Could you check a few things on this model? Use its own coordinates, in mm. Face numbers are marked on the shaded views. A direction names the side the tool comes from. Give positions to 0.01 mm unless a question says otherwise; leave off trailing zeros. Loops run counter-clockwise (first coordinate to the right, second up) from the corner with the lowest first, then second, coordinate; pieces in that order, holes last. Notation, with made-up numbers: (-14.75, -20) - (30.25, -20) arc R24 cw to (30.25, -3) - close; hole circle Ø11 at (-29, 60). An arc over 180 degrees is marked (long way). Use CSV: the item, a comma, the result in double quotes.
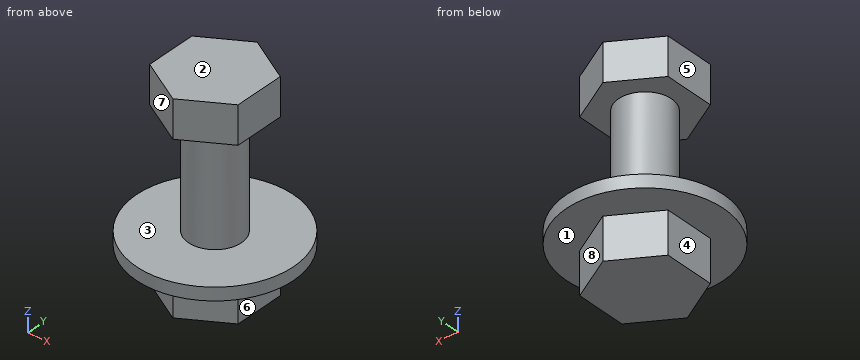
from build123d import *

# Parameters (mm, degrees)
F0_R     = 3
F1_DEPTH = 20
F3_DEPTH = 4.24
F5_DEPTH = 6
F6_R     = 8.89
F7_DEPTH = 1.4478
F9_DEPTH = 1.27


with BuildPart() as f1:
    # F0 (on Top) → F1 (new body)
    with BuildSketch(Plane.XY):
        Circle(F0_R)
    extrude(amount=-F1_DEPTH)

    # F2 (on face) → F3 (join)
    with BuildSketch(Plane.XY):
        Polygon((5, 2.8867513459), (0, 5.7735026919), (-5, 2.8867513459), (-5, -2.8867513459), (0, -5.7735026919), (5, -2.8867513459), align=None)
    extrude(amount=F3_DEPTH)

    # F4 (on face) → F5 (join)
    with BuildSketch(Plane(origin=(0, 0, -20), x_dir=(1, 0, 0), z_dir=(0, 0, -1))):
        Polygon((5, 2.8867513459), (0, 5.7735026919), (-5, 2.8867513459), (-5, -2.8867513459), (0, -5.7735026919), (5, -2.8867513459), align=None)
    extrude(amount=-F5_DEPTH)

    # F6 (on face) → F7 (join)
    with BuildSketch(Plane.XY.offset(-14)):
        Circle(F6_R)
    extrude(amount=F7_DEPTH)

    # F8 (on face) → F9 (cut)
    with BuildSketch(Plane(origin=(0, 0, -20), x_dir=(1, 0, 0), z_dir=(0, 0, -1))):
        with BuildLine():
            ThreePointArc((5, -0.8979977728), (5.0599604742, -0.4507771068), (5.08, 0))
            ThreePointArc((5.08, 0), (5.0599604742, 0.4507771068), (5, 0.8979977728))
            Line((5, 0.8979977728), (5, -0.8979977728))
        make_face()
        with BuildLine():
            Line((5, -0.8979977728), (5, 0.8979977728))
            ThreePointArc((5, 0.8979977728), (4.3994090512, 2.54), (3.2776888838, 3.8811281325))
            Line((3.2776888838, 3.8811281325), (1.7223111162, 4.7791259053))
            ThreePointArc((1.7223111162, 4.7791259053), (0, 5.08), (-1.7223111162, 4.7791259053))
            Line((-1.7223111162, 4.7791259053), (-3.2776888838, 3.8811281325))
            ThreePointArc((-3.2776888838, 3.8811281325), (-4.3994090512, 2.54), (-5, 0.8979977728))
            Line((-5, 0.8979977728), (-5, -0.8979977728))
            ThreePointArc((-5, -0.8979977728), (-4.3994090512, -2.54), (-3.2776888838, -3.8811281325))
            Line((-3.2776888838, -3.8811281325), (-1.7223111162, -4.7791259053))
            ThreePointArc((-1.7223111162, -4.7791259053), (0, -5.08), (1.7223111162, -4.7791259053))
            Line((1.7223111162, -4.7791259053), (3.2776888838, -3.8811281325))
            ThreePointArc((3.2776888838, -3.8811281325), (4.3994090512, -2.54), (5, -0.8979977728))
        make_face()
        with BuildLine():
            ThreePointArc((3.2776888838, 3.8811281325), (4.3994090512, 2.54), (5, 0.8979977728))
            Line((5, 0.8979977728), (5, 2.8867513459))
            Line((5, 2.8867513459), (3.2776888838, 3.8811281325))
        make_face()
        with BuildLine():
            Line((5, -2.8867513459), (5, -0.8979977728))
            ThreePointArc((5, -0.8979977728), (4.3994090512, -2.54), (3.2776888838, -3.8811281325))
            Line((3.2776888838, -3.8811281325), (5, -2.8867513459))
        make_face()
        with BuildLine():
            Line((1.7223111162, 4.7791259053), (3.2776888838, 3.8811281325))
            ThreePointArc((3.2776888838, 3.8811281325), (2.54, 4.3994090512), (1.7223111162, 4.7791259053))
        make_face()
        with BuildLine():
            ThreePointArc((1.7223111162, -4.7791259053), (2.54, -4.3994090512), (3.2776888838, -3.8811281325))
            Line((3.2776888838, -3.8811281325), (1.7223111162, -4.7791259053))
        make_face()
        with BuildLine():
            ThreePointArc((-1.7223111162, 4.7791259053), (0, 5.08), (1.7223111162, 4.7791259053))
            Line((1.7223111162, 4.7791259053), (0, 5.7735026919))
            Line((0, 5.7735026919), (-1.7223111162, 4.7791259053))
        make_face()
        with BuildLine():
            Line((0, -5.7735026919), (1.7223111162, -4.7791259053))
            ThreePointArc((1.7223111162, -4.7791259053), (0, -5.08), (-1.7223111162, -4.7791259053))
            Line((-1.7223111162, -4.7791259053), (0, -5.7735026919))
        make_face()
        with BuildLine():
            Line((-3.2776888838, 3.8811281325), (-1.7223111162, 4.7791259053))
            ThreePointArc((-1.7223111162, 4.7791259053), (-2.54, 4.3994090512), (-3.2776888838, 3.8811281325))
        make_face()
        with BuildLine():
            ThreePointArc((-3.2776888838, -3.8811281325), (-2.54, -4.3994090512), (-1.7223111162, -4.7791259053))
            Line((-1.7223111162, -4.7791259053), (-3.2776888838, -3.8811281325))
        make_face()
        with BuildLine():
            ThreePointArc((-5, 0.8979977728), (-4.3994090512, 2.54), (-3.2776888838, 3.8811281325))
            Line((-3.2776888838, 3.8811281325), (-5, 2.8867513459))
            Line((-5, 2.8867513459), (-5, 0.8979977728))
        make_face()
        with BuildLine():
            Line((-5, -2.8867513459), (-3.2776888838, -3.8811281325))
            ThreePointArc((-3.2776888838, -3.8811281325), (-4.3994090512, -2.54), (-5, -0.8979977728))
            Line((-5, -0.8979977728), (-5, -2.8867513459))
        make_face()
        with BuildLine():
            Line((-5, -0.8979977728), (-5, 0.8979977728))
            ThreePointArc((-5, 0.8979977728), (-5.08, 0), (-5, -0.8979977728))
        make_face()
    extrude(amount=-F9_DEPTH, mode=Mode.SUBTRACT)


solid = f1.part
1) I need wall thicknesses on line 1 along Z through (x, y) = (3.25, 1); line 2 along X through (y, z) = (1.25, 3); line 3 along Z through (x, y) = (-5.25, -3.5). Which ranges of each line are inside material? Lowest first, please.
Answer below:
line 1,"z = -18.73 to -12.55, 0 to 4.24"
line 2,"x = -5 to 5"
line 3,"z = -14 to -12.55"
2) Which directions (+Z, -Z, +X, -X, +Y, -Y) give clear straight access to the entire face, cutting with the end or side of a thin tool? Please do the marked faces 5, 6, 7 and 8.
Answer below:
face 5,"+Z, -X, +Y, -Y"
face 6,"-Z, +X, +Y, -Y"
face 7,"+Z, -X, -Y"
face 8,"-Z, +X, +Y"
3) We'd pull the mould along Z, two halves only. Please class the marked faces 1, 2, 3 and 4: +Z half, -Z half, draft (parallel to the pull), parting line (faces both ways), or undercut.
Answer below:
face 1,"-Z half"
face 2,"+Z half"
face 3,"undercut"
face 4,"draft"
4) Suppose I cut it at D-D (x = -6.75). Please give me the cut outline in (y, z).
Answer below:
outline,"(-5.79, -14) - (5.79, -14) - (5.79, -12.55) - (-5.79, -12.55) - close"
5) Suppose I cut it at B-B (z = 2.75). Please give me the cut outline in (x, y).
Answer below:
outline,"(-5, -2.89) - (0, -5.77) - (5, -2.89) - (5, 2.89) - (0, 5.77) - (-5, 2.89) - close"
6) I'm going to push flat-ended pins straight in: P1, Ø5, axis at y = 0.5, z = -17, coming from the +X side; P2, Ø3, axis at y = 1, z = -7, coming from the -X side; P3, Ø2, axis at x = -2.5, z = -11, coming from the +Y side; P4, Ø1, axis at y = 6, z = -11.5, coming from the +X side. Where does each tip first touch, or does it pass through?
Answer below:
P1,"stops at x = 5"
P2,"stops at x = -3"
P3,"stops at y = 2.6"
P4,"passes through"
7) Suppose I cut it at C-C (y = 0). Please give me the cut outline in (x, z).
Answer below:
outline,"(-8.89, -14) - (-5, -14) - (-5, -18.73) - (5, -18.73) - (5, -14) - (8.89, -14) - (8.89, -12.55) - (3, -12.55) - (3, 0) - (5, 0) - (5, 4.24) - (-5, 4.24) - (-5, 0) - (-3, 0) - (-3, -12.55) - (-8.89, -12.55) - close"
8) Suppose I cut it at A-A (y = -4.5). Please give me the cut outline in (x, z), plus the area to 3 significant figures.
Answer below:
outline,"(-7.67, -14) - (-2.21, -14) - (-2.21, -18.73) - (2.21, -18.73) - (2.21, -14) - (7.67, -14) - (7.67, -12.55) - (-7.67, -12.55) - close; (-2.21, 0) - (2.21, 0) - (2.21, 4.24) - (-2.21, 4.24) - close"
area,"61.8 mm2"
